Job drawing, mm, ordinate dimensions from the low corner. One solid piece. Coordinates: 2 decimals unless noted, no trailing zeros. Order: outer loops, then holes, each group sorted by start corner. A loop starts at its lowest first (then second) coordinate and runs counter-clockwise, first axis right, second up. Notation, with made-up numbers: M 10,87 L 39,87 A32 cw 39,113 Z; hole C 29.5,73 d11. An arc over 180 degrees is marked long. Write item = value, one per line.
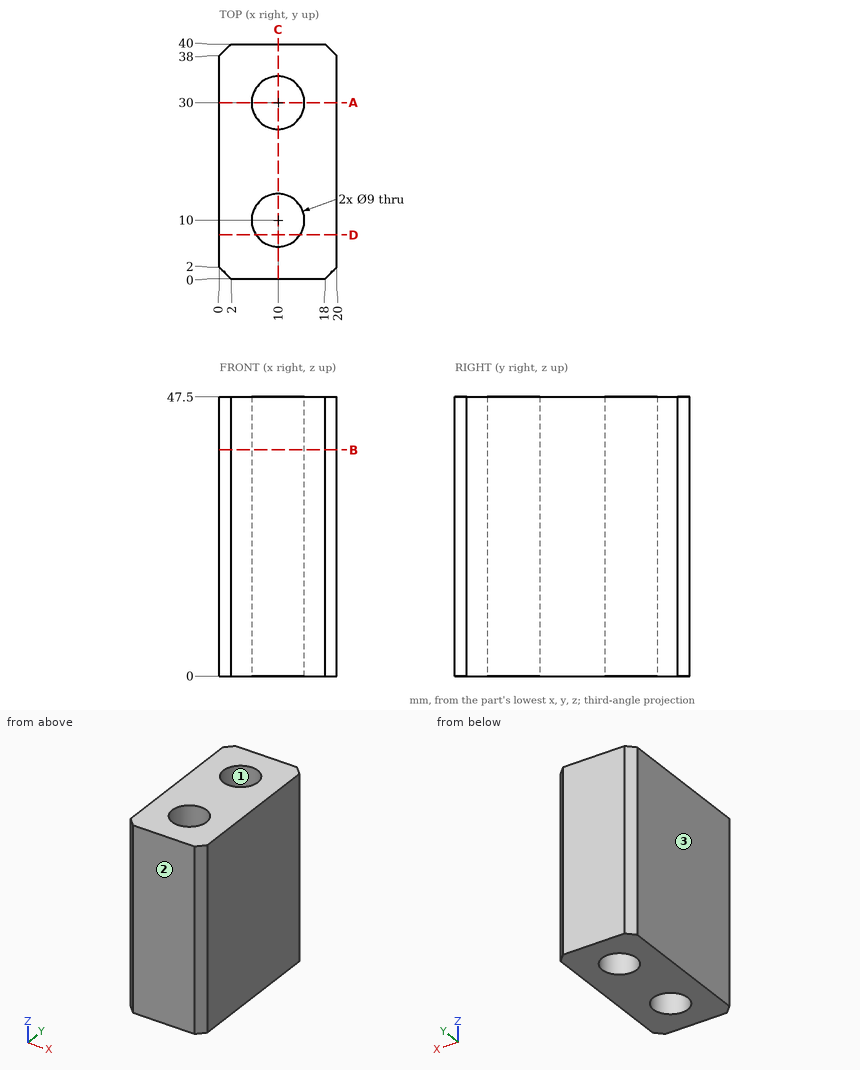
(1) Slice it at D-D, the plane y = 7.5. Write the cut outline in (x, z).
Evaluation:
outline = M 0,0 L 6.26,0 L 6.26,47.5 L 0,47.5 Z; M 13.74,0 L 20,0 L 20,47.5 L 13.74,47.5 Z
(2) Wall check: line 1 (Y direction, x = 10, z = 33.5); line 2 (Y direction, x = 8.25, z = 12); line 3 (X direction, y = 30.5, z = 7). Give the ranges that are in metal, low to high. Write a range as from..to.
Evaluation:
line_1 = 0..5.5, 14.5..25.5, 34.5..40
line_2 = 0..5.85, 14.15..25.85, 34.15..40
line_3 = 0..5.53, 14.47..20
(3) Slice it at C-C, the plane x = 10. Write the cut outline in (y, z).
Evaluation:
outline = M 0,0 L 5.5,0 L 5.5,47.5 L 0,47.5 Z; M 14.5,0 L 25.5,0 L 25.5,47.5 L 14.5,47.5 Z; M 34.5,0 L 40,0 L 40,47.5 L 34.5,47.5 Z
(4) Slice it at B-B, the plane z = 38.5. Write the cut outline in (x, y), then the cut area to 3 significant figures.
Evaluation:
outline = M 0,2 L 2,0 L 18,0 L 20,2 L 20,38 L 18,40 L 2,40 L 0,38 Z; hole C 10,10 d9; hole C 10,30 d9
area = 665 mm²
(5) Pin check, flat tip, straight feed: pin 1 Ø7 at (x, y) = (10, 30) entering from +Z. Stop position of the tip, or through.
Evaluation:
pin_1 = through
(6) Pull direction Y, two halves, no side cores. Call the marked faces 1, 2 and 3: +Y half, -Y half, draft (parallel to the pull), parting line (faces both ways), or undercut.
Evaluation:
face_1 = undercut
face_2 = -Y half
face_3 = draft
(7) Slice it at A-A, the plane y = 30. Write the cut outline in (x, z), then the cut area to 4 significant figures.
Evaluation:
outline = M 0,0 L 5.5,0 L 5.5,47.5 L 0,47.5 Z; M 14.5,0 L 20,0 L 20,47.5 L 14.5,47.5 Z
area = 522.5 mm²
